```python
from build123d import *

# Parameters (mm, degrees)
ESQUISSE1_R        = 10
BOSS_EXTRU_1_DEPTH = 52.35
BOSS_EXTRU_2_START = 6
ESQUISSE2_R        = 20
BOSS_EXTRU_2_DEPTH = 10
CONG_1_R           = 10


with BuildPart() as part:
    # Esquisse1 → Boss.-Extru.1 (new body)
    with BuildSketch(Plane.XY):
        with Locations(Location((0, 0, 0), (0, 0, 180))):
            Circle(ESQUISSE1_R)
    extrude(amount=BOSS_EXTRU_1_DEPTH)

    # Esquisse2 → Boss.-Extru.2 (add)
    with BuildSketch(Plane.XY.offset(BOSS_EXTRU_2_START)):
        Circle(ESQUISSE2_R)
    extrude(amount=BOSS_EXTRU_2_DEPTH)

    # Congé1
    cong_1_edges = [part.edges().sort_by_distance(p)[0] for p in [
        (10, 0, 16),
    ]]
    fillet(cong_1_edges, radius=CONG_1_R - 0.0001)  # a hair under: the kernel refuses the full size


solid = part.part
```
The model under review builds one solid part; all positions refer to its coordinate system, in mm. A direction names the side the tool comes from. Round coordinates to 2 decimals unless told otherwise and drop trailing zeros. Order: outer loops, then holes, each group sorted by start corner. A loop starts at its lowest first (then second) coordinate and runs counter-clockwise, first axis right, second up.
(1) Wall thickness on L1, parallel to Z at x = -13.5, y = 14.5; L2, parallel to Y at x = 14, z = 9; L3, parallel to X at y = -2, z = 44: over which ranges is each line inside the solid? List them lowest first.
Working result:
L1: z = 6 to 16
L2: y = -14.28 to 14.28
L3: x = -9.8 to 9.8
(2) Take a section at C-C, the plane z = 39.5. State the section outline as (x, y) points.
Working result:
outline: circle Ø20 at (0, 0)
(3) For P1, Ø1, axis at x = 2.5, z = 19, coming from the -Y side; P2, Ø5, axis at x = 11, z = 22.5, coming from the +Y side; P3, Ø10, axis at x = 4, z = 18, coming from the +Y side, all flat-tipped, find the tip position at first contact; note any pin that passes through.
Working result:
P1: stops at y = -13.16
P2: stops at y = 6.9
P3: stops at y = 20
(4) Take a section at D-D, the plane z = 10.5. State the section outline as (x, y) points.
Working result:
outline: circle Ø40 at (0, 0)
(5) Tool access review of faces 1 (the face through (0, 0, 0)), 2 (the face through (-5, 9, 6)), 3 (the face through (10, 0, 39)): name each direction out of +Z, -Z, +X, -X, +Y, -Y from which nothing blocks a thin tool from reaching the whole face with its end or side.
Working result:
face 1: -Z, +X, -X, +Y, -Y
face 2: -Z
face 3: +Z
